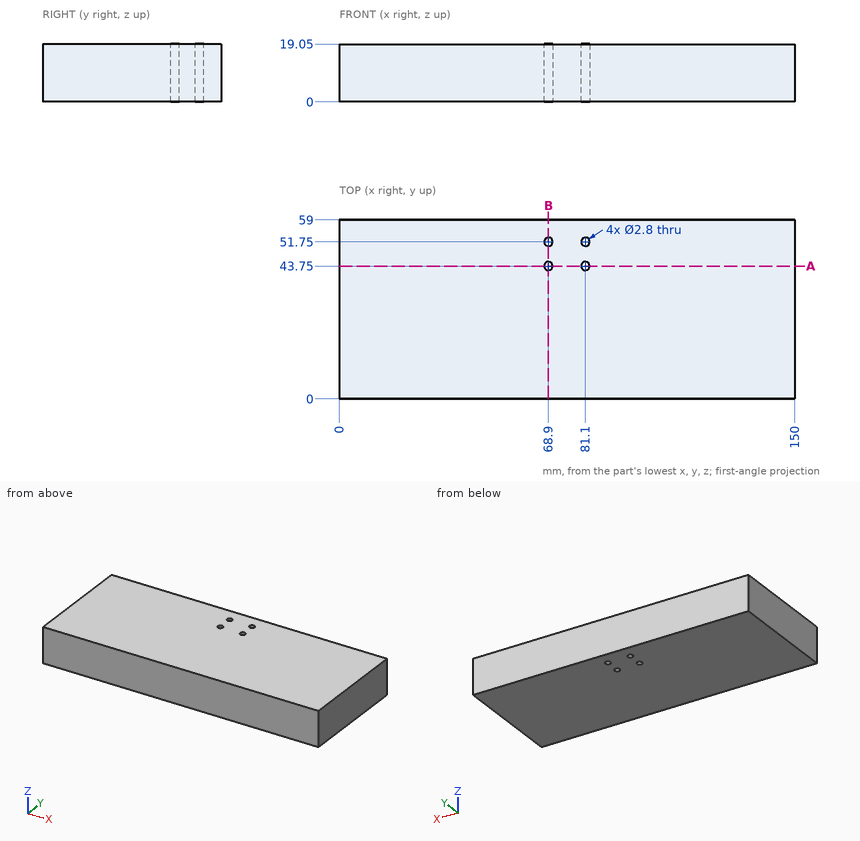
Could you check a few things on this drawing? It's one solid part, dimensions in mm from its lowest x, y, z. Coordinates: 2 decimals unless noted, no trailing zeros. Order: outer loops, then holes, each group sorted by start corner. A loop starts at its lowest first (then second) coordinate and runs counter-clockwise, first axis right, second up. Notation, with made-up numbers: M 54.25,43.25 L 100.25,43.25 A26 ccw 100.25,79.25 Z; hole C 87,86.25 d3. An arc over 180 degrees is marked long. Answer as a JSON object with one key per item and string values. Group by question number.
(1) I need wall thicknesses on probe 1 along Y at (x, z) = (68.9, 4.25); probe 2 along X at (y, z) = (44.5, 1.5). Which ranges of each line are inside material? Lowest first, please.
(2) Suppose I cut it at B-B, the plane x = 68.9. Please give me the cut outline in (y, z).
(3) Suppose I cut it at A-A, the plane y = 43.75. Please give me the cut outline in (x, z).
(4) For pin 1 (2.5 mm diameter, centred on x = 81.1, y = 51.75, fed in from -Z), with a flat end and sliding along its axis, tell me the tip position at first contact or that it passes through.
Values found:
{
 "1": {"probe 1": "y = 0 to 42.35, 45.15 to 50.35, 53.15 to 59", "probe 2": "x = 0 to 67.72, 70.08 to 79.92, 82.28 to 150"},
 "2": {"outline": "M 0,0 L 42.35,0 L 42.35,19.05 L 0,19.05 Z; M 45.15,0 L 50.35,0 L 50.35,19.05 L 45.15,19.05 Z; M 53.15,0 L 59,0 L 59,19.05 L 53.15,19.05 Z"},
 "3": {"outline": "M 0,0 L 67.5,0 L 67.5,19.05 L 0,19.05 Z; M 70.3,0 L 79.7,0 L 79.7,19.05 L 70.3,19.05 Z; M 82.5,0 L 150,0 L 150,19.05 L 82.5,19.05 Z"},
 "4": {"pin 1": "passes through"}
}
